Work out the finished part from the listing and answer in its coordinate system (mm). A direction names the side the tool comes from. Round coordinates to 2 decimals unless told otherwise and drop trailing zeros. Write each loop counter-clockwise with the first axis right and the second up, starting at its lowest first coordinate (ties: lowest second). Pieces come first, ordered by that corner, then holes. Notation, with made-up numbers: M 67.5,-24 L 71.5,-24 A15 cw 71.5,-10 Z; hole C -24.5,67 d9. An arc over 180 degrees is marked long. One line per item, written item: value. Start each with the question number.
Q1. Find section C-C (z = -8). Write down the section's boundary in (x, y), and give its area (3 significant figures).
Q2. Find section B-B (x = 35). Write down the section's boundary in (y, z), and give its area (3 significant figures).
Q3. Find section A-A (z = -5). Write down the section's boundary in (x, y), and give its area (3 significant figures).
Q4. Find section D-D (x = 11). Write down the section's boundary in (y, z).
Q5. A tool of negligible diameter and unlimited length cuts with its end or side. For faces 4 (the flat face through (19.87, 1.53, -24.28)), 5 (the flat face through (20, 5.4, -15.5)), 6 (the flat face through (20, 3, 0)), 7 (the flat face through (20, 5, -16.5)), from which of +Z, -Z, +X, -X, +Y, -Y can it reach the whole face along a straight path? Write none if from no direction.
Q6. Given pin 1 Ø2.5 at (x, z) = (5, -5) entering from -Y; pin 2 Ø6 at (x, z) = (22.5, -13) entering from -Y, each flat-ended and moving along its own axis, determine where each tip first touches the part or whether it passes through.
Q7. Consider probe 1 along X at (y, z) = (1.5, -5); probe 2 along X at (y, z) = (3.4, -25); probe 3 along Z at (x, y) = (18.5, 5). Determine where each line is inside the solid, lowest interval first.
Q8. The mould has two halves that part along Z. Classify faces 1 (the cylindrical face through (38.797, 3.042, -28.859)), 2 (the flat face through (17.5, 5, -18)), 3 (the cylindrical face through (1.141, 3.042, -1.203)): released by +Z, released by -Z, zero draft, split by the parting line, or undercut.
from build123d import *
from OCP.BRepFilletAPI import BRepFilletAPI_MakeChamfer

# Parameters (mm, degrees)
SKETCH1_W           = 40
SKETCH1_H           = 30
BOSS_EXTRUDE1_DEPTH = 6
SKETCH2_R           = 1.5
CUT_EXTRUDE1_DEPTH  = 6
FILLET1_R           = 4
SKETCH3_W           = 21
SKETCH3_H           = 21
CUT_EXTRUDE2_DEPTH  = 4
SKETCH6_W           = 5
SKETCH6_H           = 3.5
CUT_EXTRUDE3_DEPTH  = 2
SKETCH7_W           = 7
SKETCH7_H           = 5.5
SKETCH7_W_2         = 5
SKETCH7_H_2         = 3.5
BOSS_EXTRUDE2_DEPTH = 4
CHAMFER1_SIZE       = 4
CHAMFER1_SIZE2      = 6.92820323
CHAMFER2_SIZE       = 2.886751346
CHAMFER2_SIZE_2     = 5


with BuildPart() as part:
    # Sketch1 → Boss-Extrude1 (new body)
    with BuildSketch(Plane(origin=(0, 0, 0), x_dir=(1, 0, 0), z_dir=(0, 1, 0))):
        with Locations((20, 15)):
            Rectangle(SKETCH1_W, SKETCH1_H)
    extrude(amount=BOSS_EXTRUDE1_DEPTH)

    # Sketch2 → Cut-Extrude1 (cut)
    with BuildSketch(Plane(origin=(0, 6, 0), x_dir=(1, 0, 0), z_dir=(0, 1, 0))):
        with Locations(Location((5, 5, 0), (0, 0, 270))):
            Circle(SKETCH2_R)
        with Locations(Location((5, 25, 0), (0, 0, 90))):
            Circle(SKETCH2_R)
        with Locations(Location((35, 5, 0), (0, 0, 90))):
            Circle(SKETCH2_R)
        with Locations(Location((35, 25, 0), (0, 0, 270))):
            Circle(SKETCH2_R)
    extrude(amount=-CUT_EXTRUDE1_DEPTH, mode=Mode.SUBTRACT)

    # Fillet1
    fillet1_edges = [part.edges().sort_by_distance(p)[0] for p in [
        (0, 3, -30),
        (40, 3, -30),
        (40, 3, 0),
        (0, 3, 0),
    ]]
    fillet(fillet1_edges, radius=FILLET1_R)

    # Sketch3 → Cut-Extrude2 (cut)
    with BuildSketch(Plane(origin=(0, 6, 0), x_dir=(1, 0, 0), z_dir=(0, 1, 0))):
        with Locations((20, 15)):
            Rectangle(SKETCH3_W, SKETCH3_H)
    extrude(amount=-CUT_EXTRUDE2_DEPTH, mode=Mode.SUBTRACT)

    # Sketch6 → Cut-Extrude3 (cut)
    with BuildSketch(Plane(origin=(0, 2, 0), x_dir=(1, 0, 0), z_dir=(0, 1, 0))):
        with Locations((20, 18.25)):
            Rectangle(SKETCH6_W, SKETCH6_H)
    extrude(amount=-CUT_EXTRUDE3_DEPTH, mode=Mode.SUBTRACT)

    # Sketch7 → Boss-Extrude2 (add)
    with BuildSketch(Plane(origin=(0, 2, 0), x_dir=(1, 0, 0), z_dir=(0, 1, 0))):
        with Locations((20, 18.25)):
            Rectangle(SKETCH7_W, SKETCH7_H)
        with Locations((20, 18.25)):
            Rectangle(SKETCH7_W_2, SKETCH7_H_2, mode=Mode.SUBTRACT)
    extrude(amount=BOSS_EXTRUDE2_DEPTH)

    # Chamfer1: one chamfer whose edges measure the first distance from different faces: ONE call of the kernel's chamfer builder (chamfer() names one face for all edges)
    chamfer1_edges_1 = [part.edges().sort_by_distance(p)[0] for p in [
        (20, 0, -16.5),
    ]]
    chamfer1_side_1 = [part.faces().sort_by_distance(p)[0] for p in [
        (20, 3, -16.5),
    ]]
    chamfer1_edges_2 = [part.edges().sort_by_distance(p)[0] for p in [
        (22.5, 0, -18.25),
    ]]
    chamfer1_side_2 = [part.faces().sort_by_distance(p)[0] for p in [
        (22.5, 3, -18.25),
    ]]
    chamfer1_edges_3 = [part.edges().sort_by_distance(p)[0] for p in [
        (20, 0, -20),
    ]]
    chamfer1_side_3 = [part.faces().sort_by_distance(p)[0] for p in [
        (20, 3, -20),
    ]]
    chamfer1_edges_4 = [part.edges().sort_by_distance(p)[0] for p in [
        (17.5, 0, -18.25),
    ]]
    chamfer1_side_4 = [part.faces().sort_by_distance(p)[0] for p in [
        (17.5, 3, -18.25),
    ]]
    chamfer1 = BRepFilletAPI_MakeChamfer(part.part.solid().wrapped)
    for e in chamfer1_edges_1:
        chamfer1.Add(CHAMFER1_SIZE, CHAMFER1_SIZE2, e.wrapped, chamfer1_side_1[0].wrapped)  # the first distance lies on this face
    for e in chamfer1_edges_2:
        chamfer1.Add(CHAMFER1_SIZE, CHAMFER1_SIZE2, e.wrapped, chamfer1_side_2[0].wrapped)  # the first distance lies on this face
    for e in chamfer1_edges_3:
        chamfer1.Add(CHAMFER1_SIZE, CHAMFER1_SIZE2, e.wrapped, chamfer1_side_3[0].wrapped)  # the first distance lies on this face
    for e in chamfer1_edges_4:
        chamfer1.Add(CHAMFER1_SIZE, CHAMFER1_SIZE2, e.wrapped, chamfer1_side_4[0].wrapped)  # the first distance lies on this face
    add(Compound.cast(chamfer1.Shape()), mode=Mode.REPLACE)

    # Chamfer2
    # the kernel refuses this chamfer: 5, 2.886751346 mm, written as the material it adds along each edge
    with BuildSketch(Plane(origin=(16.5, 2, -33.935428773), x_dir=(0, 1, 0), z_dir=(0, 0, 1))) as chamfer2_piece_1_section:
        Polygon((CHAMFER2_SIZE, 0), (0, CHAMFER2_SIZE_2), (0, 0), align=None)
    chamfer2_piece_1 = extrude(amount=31.370857546, mode=Mode.PRIVATE)
    chamfer2_piece_1 = split(chamfer2_piece_1, bisect_by=Plane(origin=(15.883974596, 3.066987298, -33.935428773), z_dir=(-0.499999999999998, 0.8660254037844398, 0)), keep=Keep.TOP, mode=Mode.PRIVATE)
    chamfer2_piece_1 = split(chamfer2_piece_1, bisect_by=Plane(origin=(16.5, -1.436141454, -31.95157158), z_dir=(0, -0.8660254037844382, 0.500000000000001)), keep=Keep.TOP, mode=Mode.PRIVATE)
    chamfer2_piece_1 = split(chamfer2_piece_1, bisect_by=Plane(origin=(16.5, 12.147838333, -28.07657158), z_dir=(0, -0.8660254037844382, -0.500000000000001)), keep=Keep.TOP, mode=Mode.PRIVATE)
    with BuildSketch(Plane(origin=(16.5, 2, -33.935428773), x_dir=(0, 1, 0), z_dir=(0, 0, 1))) as chamfer2_piece_2_section:
        Polygon((CHAMFER2_SIZE, 0), (0, CHAMFER2_SIZE_2), (0, 0), align=None)
    chamfer2_piece_2 = extrude(amount=31.370857546, mode=Mode.PRIVATE)
    chamfer2_piece_2 = split(chamfer2_piece_2, bisect_by=Plane(origin=(16.5, -2.534217665, -31.317596984), z_dir=(0, 0.8660254037844398, -0.499999999999998)), keep=Keep.TOP, mode=Mode.PRIVATE)
    chamfer2_piece_2 = split(chamfer2_piece_2, bisect_by=Plane(origin=(16.5, -1.436141454, -31.95157158), z_dir=(0, -0.8660254037844382, 0.500000000000001)), keep=Keep.TOP, mode=Mode.PRIVATE)
    with BuildSketch(Plane(origin=(16.5, 2, -33.935428773), x_dir=(0, 1, 0), z_dir=(0, 0, 1))) as chamfer2_piece_3_section:
        Polygon((CHAMFER2_SIZE, 0), (0, CHAMFER2_SIZE_2), (0, 0), align=None)
    chamfer2_piece_3 = extrude(amount=31.370857546, mode=Mode.PRIVATE)
    chamfer2_piece_3 = split(chamfer2_piece_3, bisect_by=Plane(origin=(16.5, 11.049762122, -28.710546176), z_dir=(0, 0.8660254037844398, 0.499999999999998)), keep=Keep.TOP, mode=Mode.PRIVATE)
    chamfer2_piece_3 = split(chamfer2_piece_3, bisect_by=Plane(origin=(16.5, 12.147838333, -28.07657158), z_dir=(0, -0.8660254037844382, -0.500000000000001)), keep=Keep.TOP, mode=Mode.PRIVATE)
    with BuildSketch(Plane(origin=(3.564571227, 2, -15.5), x_dir=(0, 1, 0), z_dir=(1, 0, 0))) as chamfer2_piece_4_section:
        Polygon((CHAMFER2_SIZE, 0), (0, CHAMFER2_SIZE_2), (0, 0), align=None)
    chamfer2_piece_4 = extrude(amount=32.870857546, mode=Mode.PRIVATE)
    chamfer2_piece_4 = split(chamfer2_piece_4, bisect_by=Plane(origin=(3.564571227, 3.066987298, -14.883974596), z_dir=(0, 0.8660254037844398, 0.499999999999998)), keep=Keep.TOP, mode=Mode.PRIVATE)
    chamfer2_piece_4 = split(chamfer2_piece_4, bisect_by=Plane(origin=(9.79842842, 12.797357386, -15.5), z_dir=(-0.500000000000001, -0.8660254037844382, 0)), keep=Keep.TOP, mode=Mode.PRIVATE)
    chamfer2_piece_4 = split(chamfer2_piece_4, bisect_by=Plane(origin=(5.54842842, -1.436141454, -15.5), z_dir=(0.500000000000001, -0.8660254037844382, 0)), keep=Keep.TOP, mode=Mode.PRIVATE)
    with BuildSketch(Plane(origin=(3.564571227, 2, -15.5), x_dir=(0, 1, 0), z_dir=(1, 0, 0))) as chamfer2_piece_5_section:
        Polygon((CHAMFER2_SIZE, 0), (0, CHAMFER2_SIZE_2), (0, 0), align=None)
    chamfer2_piece_5 = extrude(amount=32.870857546, mode=Mode.PRIVATE)
    chamfer2_piece_5 = split(chamfer2_piece_5, bisect_by=Plane(origin=(6.182403016, -2.534217665, -15.5), z_dir=(-0.499999999999998, 0.8660254037844398, 0)), keep=Keep.TOP, mode=Mode.PRIVATE)
    chamfer2_piece_5 = split(chamfer2_piece_5, bisect_by=Plane(origin=(5.54842842, -1.436141454, -15.5), z_dir=(0.500000000000001, -0.8660254037844382, 0)), keep=Keep.TOP, mode=Mode.PRIVATE)
    with BuildSketch(Plane(origin=(23.5, 2, -2.564571227), x_dir=(0, 1, 0), z_dir=(0, 0, -1))) as chamfer2_piece_6_section:
        Polygon((CHAMFER2_SIZE, 0), (0, CHAMFER2_SIZE_2), (0, 0), align=None)
    chamfer2_piece_6 = extrude(amount=31.370857546, mode=Mode.PRIVATE)
    chamfer2_piece_6 = split(chamfer2_piece_6, bisect_by=Plane(origin=(24.116025404, 3.066987298, -2.564571227), z_dir=(0.499999999999998, 0.8660254037844398, 0)), keep=Keep.TOP, mode=Mode.PRIVATE)
    chamfer2_piece_6 = split(chamfer2_piece_6, bisect_by=Plane(origin=(23.5, 12.147838333, -8.42342842), z_dir=(0, -0.8660254037844382, 0.500000000000001)), keep=Keep.TOP, mode=Mode.PRIVATE)
    chamfer2_piece_6 = split(chamfer2_piece_6, bisect_by=Plane(origin=(23.5, -1.436141454, -4.54842842), z_dir=(0, -0.8660254037844382, -0.500000000000001)), keep=Keep.TOP, mode=Mode.PRIVATE)
    with BuildSketch(Plane(origin=(23.5, 2, -2.564571227), x_dir=(0, 1, 0), z_dir=(0, 0, -1))) as chamfer2_piece_7_section:
        Polygon((CHAMFER2_SIZE, 0), (0, CHAMFER2_SIZE_2), (0, 0), align=None)
    chamfer2_piece_7 = extrude(amount=31.370857546, mode=Mode.PRIVATE)
    chamfer2_piece_7 = split(chamfer2_piece_7, bisect_by=Plane(origin=(23.5, -2.534217665, -5.182403016), z_dir=(0, 0.8660254037844398, 0.499999999999998)), keep=Keep.TOP, mode=Mode.PRIVATE)
    chamfer2_piece_7 = split(chamfer2_piece_7, bisect_by=Plane(origin=(23.5, -1.436141454, -4.54842842), z_dir=(0, -0.8660254037844382, -0.500000000000001)), keep=Keep.TOP, mode=Mode.PRIVATE)
    with BuildSketch(Plane(origin=(23.5, 2, -2.564571227), x_dir=(0, 1, 0), z_dir=(0, 0, -1))) as chamfer2_piece_8_section:
        Polygon((CHAMFER2_SIZE, 0), (0, CHAMFER2_SIZE_2), (0, 0), align=None)
    chamfer2_piece_8 = extrude(amount=31.370857546, mode=Mode.PRIVATE)
    chamfer2_piece_8 = split(chamfer2_piece_8, bisect_by=Plane(origin=(23.5, 11.049762122, -7.789453824), z_dir=(0, 0.8660254037844398, -0.499999999999998)), keep=Keep.TOP, mode=Mode.PRIVATE)
    chamfer2_piece_8 = split(chamfer2_piece_8, bisect_by=Plane(origin=(23.5, 12.147838333, -8.42342842), z_dir=(0, -0.8660254037844382, 0.500000000000001)), keep=Keep.TOP, mode=Mode.PRIVATE)
    with BuildSketch(Plane(origin=(36.435428773, 2, -21), x_dir=(0, 1, 0), z_dir=(-1, 0, 0))) as chamfer2_piece_9_section:
        Polygon((CHAMFER2_SIZE, 0), (0, CHAMFER2_SIZE_2), (0, 0), align=None)
    chamfer2_piece_9 = extrude(amount=32.870857546, mode=Mode.PRIVATE)
    chamfer2_piece_9 = split(chamfer2_piece_9, bisect_by=Plane(origin=(36.435428773, 3.066987298, -21.616025404), z_dir=(0, 0.8660254037844398, -0.499999999999998)), keep=Keep.TOP, mode=Mode.PRIVATE)
    chamfer2_piece_9 = split(chamfer2_piece_9, bisect_by=Plane(origin=(34.45157158, -1.436141454, -21), z_dir=(-0.500000000000001, -0.8660254037844382, 0)), keep=Keep.TOP, mode=Mode.PRIVATE)
    chamfer2_piece_9 = split(chamfer2_piece_9, bisect_by=Plane(origin=(30.20157158, 12.797357386, -21), z_dir=(0.500000000000001, -0.8660254037844382, 0)), keep=Keep.TOP, mode=Mode.PRIVATE)
    with BuildSketch(Plane(origin=(36.435428773, 2, -21), x_dir=(0, 1, 0), z_dir=(-1, 0, 0))) as chamfer2_piece_10_section:
        Polygon((CHAMFER2_SIZE, 0), (0, CHAMFER2_SIZE_2), (0, 0), align=None)
    chamfer2_piece_10 = extrude(amount=32.870857546, mode=Mode.PRIVATE)
    chamfer2_piece_10 = split(chamfer2_piece_10, bisect_by=Plane(origin=(30.835546176, 11.699281175, -21), z_dir=(-0.499999999999998, 0.8660254037844398, 0)), keep=Keep.TOP, mode=Mode.PRIVATE)
    chamfer2_piece_10 = split(chamfer2_piece_10, bisect_by=Plane(origin=(30.20157158, 12.797357386, -21), z_dir=(0.500000000000001, -0.8660254037844382, 0)), keep=Keep.TOP, mode=Mode.PRIVATE)
    add([chamfer2_piece_1, chamfer2_piece_2, chamfer2_piece_3, chamfer2_piece_4, chamfer2_piece_5, chamfer2_piece_6, chamfer2_piece_7, chamfer2_piece_8, chamfer2_piece_9, chamfer2_piece_10])


solid = part.part
The answers:
1. outline: M 0,0 L 40,0 L 40,6 L 30.5,6 L 30.5,2 L 9.5,2 L 9.5,6 L 0,6 Z
1. area: 156 mm2
2. outline: M 0,-30 L 6,-30 L 6,-26.5 L 0,-26.5 Z; M 0,-23.5 L 6,-23.5 L 6,-6.5 L 0,-6.5 Z; M 0,-3.5 L 6,-3.5 L 6,0 L 0,0 Z
2. area: 144 mm2
3. outline: M 0,0 L 3.5,0 L 3.5,6 L 0,6 Z; M 6.5,0 L 33.5,0 L 33.5,6 L 30.5,6 L 30.5,2 L 9.5,2 L 9.5,6 L 6.5,6 Z; M 36.5,0 L 40,0 L 40,6 L 36.5,6 Z
3. area: 120 mm2
4. outline: M 0,-30 L 6,-30 L 6,-25.5 L 2,-25.5 L 2,-4.5 L 6,-4.5 L 6,0 L 0,0 L 0,-9.57 L 0.25,-10 L 0.25,-26.5 L 0,-26.93 Z
5. face 4: -Y
5. face 5: +Y
5. face 6: +Z, +X, -X, +Y, -Y
5. face 7: +Y, -Y
6. pin 1: through
6. pin 2: y = 0.25
7. probe 1: 0 to 3.5, 6.5 to 33.5, 36.5 to 40
7. probe 2: 0 to 3.5, 6.5 to 9.5, 30.5 to 33.5, 36.5 to 40
7. probe 3: -30 to -25.5, -21 to -20, -16.5 to -15.5, -4.5 to 0
8. face 1: released by -Z
8. face 2: undercut
8. face 3: released by +Z
